```python
from build123d import *

# Parameters (mm, degrees)
EXTRUDE_3_DEPTH     = 10
SKETCH_5_W          = 19
SKETCH_5_H          = 3
EXTRUDE_5_DEPTH     = 19
SKETCH_6_R          = 1.6
CUT_EXTRUDE_4_DEPTH = 19
SKETCH_7_W          = 19
SKETCH_7_H          = 19
CUT_EXTRUDE_5_DEPTH = 0.5
SKETCH_8_W          = 19
SKETCH_8_H          = 19
CUT_EXTRUDE_7_DEPTH = 0.5


with BuildPart() as part:
    # 草图1 → 凸台-拉伸3 (new body)
    with BuildSketch(Plane(origin=(0, 0, 0), x_dir=(1, 0, 0), z_dir=(0, 1, 0))):
        Polygon((-7.404411765, -8.672794118), (-5.404411765, -8.672794118), (-5.404411765, -10.672794118), (-9.404411765, -10.672794118), (-9.404411765, 8.327205882), (9.595588235, 8.327205882), (9.595588235, -10.672794118), (5.595588235, -10.672794118), (5.595588235, -8.672794118), (7.595588235, -8.672794118), (7.595588235, 6.327205882), (-7.404411765, 6.327205882), align=None)
    extrude(amount=EXTRUDE_3_DEPTH)

    # 草图5 → 凸台-拉伸5 (add)
    with BuildSketch(Plane(origin=(9.595588235, 0, 0), x_dir=(0, 0, -1), z_dir=(1, 0, 0))):
        with Locations((-1.172794118, 8.5)):
            Rectangle(SKETCH_5_W, SKETCH_5_H)
        with Locations((-1.172794118, 1.5)):
            Rectangle(SKETCH_5_W, SKETCH_5_H)
    extrude(amount=EXTRUDE_5_DEPTH)

    # 草图6 → 切除-拉伸4 (cut)
    with BuildSketch(Plane.XZ):
        with Locations(Location((19.095588235, 1.172794118, 0), (0, 0, 270))):
            Circle(SKETCH_6_R)
        with BuildLine():
            Line((23.595588235, 10.672794118), (28.595588235, 10.672794118))
            Line((28.595588235, 10.672794118), (28.595588235, 5.672794118))
            ThreePointArc((28.595588235, 5.672794118), (27.131122141, 9.208328024), (23.595588235, 10.672794118))
        make_face()
        with BuildLine():
            Line((28.595588235, -3.327205882), (28.595588235, -8.327205882))
            Line((28.595588235, -8.327205882), (23.595588235, -8.327205882))
            ThreePointArc((23.595588235, -8.327205882), (27.131122141, -6.862739788), (28.595588235, -3.327205882))
        make_face()
    extrude(amount=-CUT_EXTRUDE_4_DEPTH, mode=Mode.SUBTRACT)

    # 草图7 → 切除-拉伸5 (cut)
    with BuildSketch(Plane.XZ.offset(-7)):
        with Locations((19.095588235, 1.172794118)):
            Rectangle(SKETCH_7_W, SKETCH_7_H)
    extrude(amount=-CUT_EXTRUDE_5_DEPTH, mode=Mode.SUBTRACT)

    # 草图8 → 切除-拉伸7 (cut)
    with BuildSketch(Plane(origin=(0, 3, 0), x_dir=(1, 0, 0), z_dir=(0, 1, 0))):
        with Locations((19.095588235, -1.172794118)):
            Rectangle(SKETCH_8_W, SKETCH_8_H)
    extrude(amount=-CUT_EXTRUDE_7_DEPTH, mode=Mode.SUBTRACT)


solid = part.part
```
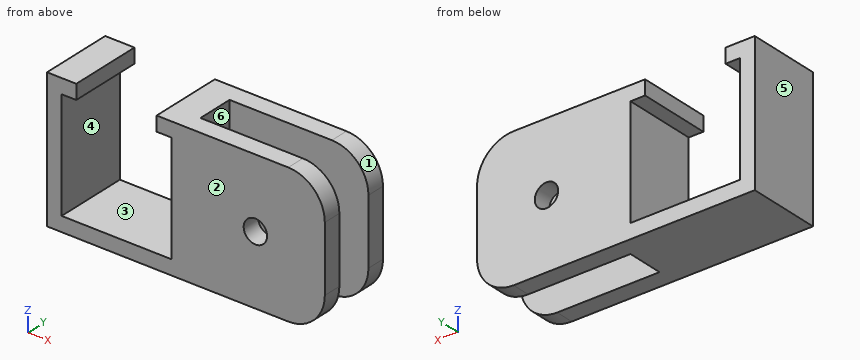
Read the model definition and answer for the solid it produces. Units are mm, in the model's axes. Face numbers are marked on the shaded views. A direction names the side the tool comes from. Round coordinates to 2 decimals unless told otherwise and drop trailing zeros. Write each loop counter-clockwise with the first axis right and the second up, starting at its lowest first coordinate (ties: lowest second). Pieces come first, ordered by that corner, then holes. Notation, with made-up numbers: M -33,67.5 L -7,67.5 A21 ccw -7,86.5 Z; hole C -20.75,-39 d5. An arc over 180 degrees is marked long. One line per item, written item: value.
Q1. Find section A-A on x = 10. Write down the section's boundary in (y, z), plus the area to 3 significant figures.
Data:
outline: M 0,-8.33 L 2.5,-8.33 L 2.5,10.67 L 0,10.67 Z; M 7.5,-8.33 L 10,-8.33 L 10,10.67 L 7.5,10.67 Z
area: 95.0 mm2
Q2. Find section D-D on z = 2. Write down the section's boundary in (x, y).
Data:
outline: M -9.4,0 L -7.4,0 L -7.4,10 L -9.4,10 Z; M 7.6,0 L 17.73,0 L 17.73,2.5 L 9.6,2.5 L 9.6,7.5 L 17.73,7.5 L 17.73,10 L 7.6,10 Z; M 20.47,0 L 28.6,0 L 28.6,2.5 L 20.47,2.5 Z; M 20.47,7.5 L 28.6,7.5 L 28.6,10 L 20.47,10 Z
Q3. For a pull along Z with two mould halves and no side action, classify the marked faces 1, 2 and 3 as +Z half, -Z half, draft (parallel to the pull), parting line (faces both ways), or undercut.
Data:
face 1: +Z half
face 2: draft
face 3: undercut
Q4. Find section B-B on z = -2.25. Write down the section's boundary in (x, y), plus the area to 3 significant figures.
Data:
outline: M -9.4,0 L -7.4,0 L -7.4,10 L -9.4,10 Z; M 7.6,0 L 28.6,0 L 28.6,2.5 L 9.6,2.5 L 9.6,7.5 L 28.6,7.5 L 28.6,10 L 7.6,10 Z
area: 135 mm2
Q5. Find section C-C on y = 3.5. Write down the section's boundary in (x, z), plus the area to 3 significant figures.
Data:
outline: M -9.4,-8.33 L 9.6,-8.33 L 9.6,10.67 L 5.6,10.67 L 5.6,8.67 L 7.6,8.67 L 7.6,-6.33 L -7.4,-6.33 L -7.4,8.67 L -5.4,8.67 L -5.4,10.67 L -9.4,10.67 Z
area: 114 mm2
Q6. Straight lines are drawn through the part: line 1 (X direction, y = 6.5, z = 5.5); line 2 (Y direction, x = 18.5, z = -3.5); line 3 (X direction, y = 0.5, z = -0.75). For each, find the intervals that lie inside material, in ascending order. Write a range as [from, to].
Data:
line 1: [-9.4, -7.4], [7.6, 9.6]
line 2: [0, 2.5], [7.5, 10]
line 3: [-9.4, -7.4], [7.6, 28.6]
Q7. Which of the six approach directions +Z, -Z, +X, -X, +Y, -Y give full straight-line access (tool end or side, diameter ignored) to the marked faces 4, 5 and 6?
Data:
face 4: +Y, -Y
face 5: +Z, -Z, -X, +Y, -Y
face 6: +Z, -Z, +X
Q8. Flat-ended cylindrical pins translate along their axes: pin 1 Ø9.5 at (x, z) = (20, 3.5) entering from -Y; pin 2 Ø3 at (x, y) = (0.5, 3) entering from +Z; pin 3 Ø0.6 at (y, z) = (4, 9.5) entering from +X. Find the tip coordinate at first contact, or state that the pin passes through.
Data:
pin 1: y = 0
pin 2: z = -6.33
pin 3: x = 9.6
